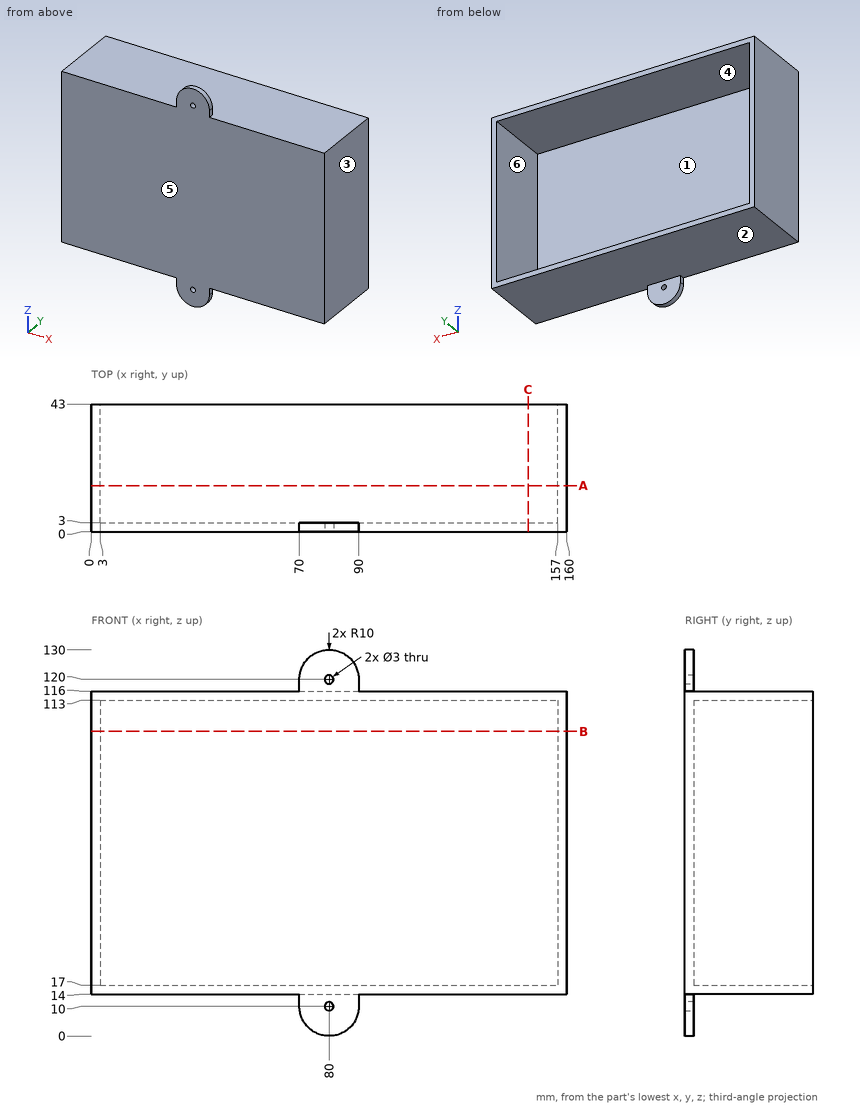
Source: three-view drawing plus pictorial views. Frame: mm from the lowest corner of the part. A direction names the side the tool comes from. Coordinates: 2 decimals unless noted, no trailing zeros. Order: outer loops, then holes, each group sorted by start corner. A loop starts at its lowest first (then second) coordinate and runs counter-clockwise, first axis right, second up. Notation, with made-up numbers: M -6,75 L 34,75 A21 ccw 34,91 Z; hole C 46,83.5 d9. An arc over 180 degrees is marked long. One line per question, with ' | ' between items.
Item 1: Draft query along X for the marked faces 1, 2, 3 and 4. Return one class per face: released by +X, released by -X, zero draft, split by the parting line, or undercut.
Geometry results:
face 1: undercut | face 2: zero draft | face 3: released by +X | face 4: undercut
Item 2: Reachability of the marked faces 5 and 6 from +Z, -Z, +X, -X, +Y, -Y: full face, straight path, thin tool, end or side. Return the list, or none.
Geometry results:
face 5: +Z, -Z, +X, -X, -Y | face 6: +Y
Item 3: Section C-C (x = 147). Output: boundary loops of the cut face in (y, z), then the cut area to 3 significant figures.
Geometry results:
outline: M 0,14 L 43,14 L 43,17 L 3,17 L 3,113 L 43,113 L 43,116 L 0,116 Z | area: 546 mm^2
Item 4: Section A-A (y = 15.5). Output: boundary loops of the cut face in (x, z).
Geometry results:
outline: M 0,14 L 160,14 L 160,116 L 0,116 Z; hole M 3,17 L 157,17 L 157,113 L 3,113 Z
Item 5: Section B-B (z = 102.5). Output: boundary loops of the cut face in (x, y), then the cut area to 3 significant figures.
Geometry results:
outline: M 0,0 L 160,0 L 160,43 L 157,43 L 157,3 L 3,3 L 3,43 L 0,43 Z | area: 720 mm^2
Item 6: Pin query (flat end, axial travel): pin 1 (1 mm diameter, centred on x = 110, z = 25, fed in from +Y); pin 2 (3.5 mm diameter, centred on y = 1, z = 12, fed in from +X); pin 3 (0.9 mm diameter, centred on y = 1, z = 11.5, fed in from -X); pin 4 (6 mm diameter, centred on x = 96.5, z = 114, fed in from -Y). Return the tip coordinate at first contact, or that it passes through.
Geometry results:
pin 1: stops at y = 3 | pin 2: stops at x = 90 | pin 3: stops at x = 70 | pin 4: stops at y = 0
Item 7: Ray query, line 1 along Z through (x, y) = (12, 23); line 2 along X through (y, z) = (1, 120); line 3 along X through (y, z) = (17.5, 53). Return the intervals inside material, ascending.
Geometry results:
line 1: z = 14 to 17, 113 to 116 | line 2: x = 70 to 78.5, 81.5 to 90 | line 3: x = 0 to 3, 157 to 160
